```python
from build123d import *

# Parameters (mm, degrees)
BOSS_EXTRUDE1_DEPTH = 30
SKETCH2_R           = 11.35
BOSS_EXTRUDE2_DEPTH = 35
SKETCH3_R           = 3.7
CUT_EXTRUDE1_DEPTH  = 75.22257831
CUT_EXTRUDE2_DEPTH  = 28


with BuildPart() as part:
    # Sketch1 → Boss-Extrude1 (new body)
    with BuildSketch(Plane.XY):
        with BuildLine():
            Line((-31.808576883, -15.32365322), (31.808576883, -15.32365322))
            Line((31.808576883, -15.32365322), (31.808576883, -4.32365322))
            Line((31.808576883, -4.32365322), (15.808576883, -4.32365322))
            add(Edge.make_bspline(
                [(12.175, 0), (12.801032904, -3.083922052), (15.808576883, -4.32365322)],
                knots=[0, 0, 0, 1, 1, 1], degree=2))
            ThreePointArc((12.175, 0), (0, 12.175), (-12.175, 0))
            add(Edge.make_bspline(
                [(-12.175, 0), (-12.801032904, -3.083922052), (-15.808576883, -4.32365322)],
                knots=[0, 0, 0, 1, 1, 1], degree=2))
            Line((-15.808576883, -4.32365322), (-31.808576883, -4.32365322))
            Line((-31.808576883, -4.32365322), (-31.808576883, -15.32365322))
        make_face()
    extrude(amount=BOSS_EXTRUDE1_DEPTH)

    # Sketch2 → Boss-Extrude2 (add)
    with BuildSketch(Plane.XY.offset(30)):
        Circle(SKETCH2_R)
    extrude(amount=BOSS_EXTRUDE2_DEPTH)

    # Sketch3 → Cut-Extrude1 (cut, through all)
    with BuildSketch(Plane(origin=(0, -4.32365322, 0), x_dir=(1, 0, 0), z_dir=(0, 1, 0))):
        with Locations(Location((-23.808576883, -7.5, 0), (0, 0, 270))):
            Circle(SKETCH3_R)
        with Locations(Location((-23.808576883, -22.5, 0), (0, 0, 90))):
            Circle(SKETCH3_R)
        with Locations(Location((23.808576883, -22.5, 0), (0, 0, 270))):
            Circle(SKETCH3_R)
        with Locations(Location((23.808576883, -7.5, 0), (0, 0, 90))):
            Circle(SKETCH3_R)
    extrude(amount=-CUT_EXTRUDE1_DEPTH, mode=Mode.SUBTRACT)

    # Sketch5 → Cut-Extrude2 (cut)
    with BuildSketch(Plane.XY.offset(65)):
        Polygon((-3.75, -11.35), (3.75, -11.35), (6, -11.35), (6, -0.35), (-6, -0.35), (-6, -11.35), align=None)
    extrude(amount=-CUT_EXTRUDE2_DEPTH, mode=Mode.SUBTRACT)


solid = part.part
```
Model file for the job. Use its own axes, mm. A direction names the side the tool comes from. Round coordinates to 2 decimals unless told otherwise and drop trailing zeros. Write each loop counter-clockwise with the first axis right and the second up, starting at its lowest first coordinate (ties: lowest second). Pieces come first, ordered by that corner, then holes. Notation, with made-up numbers: (50, -34) - (104, -34) arc R18 ccw to (104, -4) - close; hole circle Ø3 at (62, 21). An arc over 180 degrees is marked (long way). One line per item, written item: value.
(1) Cut at A-A, the plane y = -8.5. Give the cut face in (x, z), plus the area to 3 significant figures.
Values follow:
outline: (-31.81, 0) - (31.81, 0) - (31.81, 30) - (7.52, 30) - (7.52, 65) - (6, 65) - (6, 37) - (-6, 37) - (-6, 65) - (-7.52, 65) - (-7.52, 30) - (-31.81, 30) - close; hole circle Ø7.4 at (-23.81, 7.5); hole circle Ø7.4 at (-23.81, 22.5); hole circle Ø7.4 at (23.81, 7.5); hole circle Ø7.4 at (23.81, 22.5)
area: 1,930 mm²
(2) Wall check: probe 1 along X at (y, z) = (-11.5, 22.5); probe 2 along Z at (x, y) = (-21, -12.75); probe 3 along Z at (x, y) = (-4, -7.75). Give the ranges that are in metal, low to high.
Values follow:
probe 1: x = -31.81 to -27.51, -20.11 to 20.11, 27.51 to 31.81
probe 2: z = 0 to 5.09, 9.91 to 20.09, 24.91 to 30
probe 3: z = 0 to 37
(3) Cut at B-B, the plane x = 0. Give the cut face in (y, z) (3 decimals).
Values follow:
outline: (-15.324, 0) - (12.175, 0) - (12.175, 30) - (11.35, 30) - (11.35, 65) - (-0.35, 65) - (-0.35, 37) - (-11.35, 37) - (-11.35, 30) - (-15.324, 30) - close
(4) Cut at C-C, the plane z = 7.5. Give the number of separate pieces and of enclosed holes in the cut face, plus the area to 3 significant figures.
Values follow:
separate pieces: 3
enclosed holes: 0
area: 885 mm²
(5) 3-axis set-ups, long thin cutter, end or side, ignore diameter. For faces 1 (the flat face through (24, -4.324, 15)), 2 (the flat face through (-24, -4.324, 15)), 3 (the flat face through (-31.809, -10, 15)), 4 (the flat face through (-6, -5, 51)): which of +Z, -Z, +X, -X, +Y, -Y reach the whole face in a straight line?
Values follow:
face 1: +Z, -Z, +X, +Y
face 2: +Z, -Z, -X, +Y
face 3: +Z, -Z, -X, +Y, -Y
face 4: +Z, -Y
(6) Drop flat-ended pins along their axis: P1, Ø6, axis at x = 7, z = 19, coming from the +Y side; P2, Ø6.5, axis at x = 23.81, z = 22.5, coming from the -Y side; P3, Ø17.5, axis at x = -22.5, z = 17.5, coming from the +Y side; P4, Ø12, axis at x = 23.81, z = 7.5, coming from the +Y side. Give the stop position or say it passes through.
Values follow:
P1: stops at y = 11.5
P2: passes through
P3: stops at y = -3
P4: stops at y = -4.32
(7) Cut at D-D, the plane y = 5. Give the cut face in (x, z), plus the area to 3 significant figures.
Values follow:
outline: (-11.1, 0) - (11.1, 0) - (11.1, 30) - (10.19, 30) - (10.19, 65) - (-10.19, 65) - (-10.19, 30) - (-11.1, 30) - close
area: 1,380 mm²
(8) Two-plate mould, pull along X, no slides. Class faces 5 (the cylindrical face through (20.14, -9.75, 7.98)), 6 (the flat face through (0, -15.324, 15)), 7 (the cylindrical face through (-1.478, 11.253, 47.255)), 8 (the flat face through (31.809, -10, 15)): pulls with the +X half, pulls with the -X half, needs draft (parallel to the pull), parting line crosses it, or undercut.
Values follow:
face 5: undercut
face 6: needs draft
face 7: parting line crosses it
face 8: pulls with the +X half
